```python
from build123d import *

# Parameters (mm, degrees)
F1_DEPTH = 12.7
F4_D     = 13.4874
F5_D     = 25.654


with BuildPart() as f1:
    # F0 (on Front) → F1 (new body)
    with BuildSketch(Plane.XZ):
        with BuildLine():
            Line((-19.05, 50.8), (19.05, 50.8))
            ThreePointArc((19.05, 50.8), (0, 69.85), (-19.05, 50.8))
        make_face()
        with BuildLine():
            ThreePointArc((-19.05, 50.8), (0, 31.75), (19.05, 50.8))
            Line((19.05, 50.8), (-19.05, 50.8))
        make_face()
        with BuildLine():
            ThreePointArc((-19.05, 0), (0, 19.05), (19.05, 0))
            Line((19.05, 0), (19.05, 50.8))
            ThreePointArc((19.05, 50.8), (0, 31.75), (-19.05, 50.8))
            Line((-19.05, 50.8), (-19.05, 0))
        make_face()
        with BuildLine():
            Line((-19.05, 0), (19.05, 0))
            ThreePointArc((19.05, 0), (0, 19.05), (-19.05, 0))
        make_face()
        with BuildLine():
            ThreePointArc((-19.05, 0), (0, -19.05), (19.05, 0))
            Line((19.05, 0), (-19.05, 0))
        make_face()
    extrude(amount=F1_DEPTH)

    # F4 (through all)
    with Locations(Plane.XZ.offset(12.7)):
        with Locations((0, 50.8)):
            Hole(F4_D / 2)

    # F5 (through all)
    with Locations(Plane.XZ.offset(12.7)):
        with Locations((0, 0)):
            Hole(F5_D / 2)


solid = f1.part
```
The listing builds one solid part. Answer for the finished solid, in the listing's coordinates (mm). Give positions to 0.01 mm unless a question says otherwise; leave off trailing zeros. Loops run counter-clockwise (first coordinate to the right, second up) from the corner with the lowest first, then second, coordinate; pieces in that order, holes last. Notation, with made-up numbers: M 80.25,8.25 L 100.25,8.25 A16 ccw 100.25,23.25 Z; hole C -11.75,-27 d11. An arc over 180 degrees is marked long. One line per item, written item: value.
1. Section D-D on x = 9 is taken. Determine the outline of the cut face in (y, z), plus the area to 3 significant figures.
Found:
outline: M -12.7,-16.79 L 0,-16.79 L 0,-9.14 L -12.7,-9.14 Z; M -12.7,9.14 L 0,9.14 L 0,67.59 L -12.7,67.59 Z
area: 839 mm^2
2. Section C-C on z = 3 is taken. Determine the outline of the cut face in (x, y).
Found:
outline: M -19.05,-12.7 L -12.47,-12.7 L -12.47,0 L -19.05,0 Z; M 12.47,-12.7 L 19.05,-12.7 L 19.05,0 L 12.47,0 Z
3. Each of these flat-tipped pins is pushed along its axis until it touches: P1, Ø2, axis at x = -12, y = -10, coming from the +Z side; P2, Ø4, axis at x = 15, y = -5, coming from the +Z side; P3, Ø6, axis at x = -12.5, y = -7, coming from the -Z side. Where does it stop, or does it pass through?
Found:
P1: z = 66.35
P2: z = 64.72
P3: z = -16.51
4. Find the intervals of material crossed by probe 1 along Z at (x, y) = (0.5, -2.5); probe 2 along Z at (x, y) = (3, -10); probe 3 along Z at (x, y) = (-7.5, -8), in increasing order.
Found:
probe 1: -19.04 to -12.82, 12.82 to 44.07, 57.53 to 69.84
probe 2: -18.81 to -12.47, 12.47 to 44.76, 56.84 to 69.61
probe 3: -17.51 to -10.41, 10.41 to 68.31
5. For a pull along Z with two mould halves and no side action, classify faces 1 (the face through (-0.419, -6.261, -19.045)), 2 (the face through (-12.235, -6.261, 3.853)), 3 (the face through (0.878, -6.261, 57.486)), 4 (the face through (0, -12.7, 26)) as pulls with the +Z half, pulls with the -Z half, needs draft (parallel to the pull), parting line crosses it, or undercut.
Found:
face 1: pulls with the -Z half
face 2: undercut
face 3: undercut
face 4: needs draft
6. Section B-B on y = -1.75 is taken. Determine the outline of the cut face in (x, z).
Found:
outline: M -19.05,0 A19.05 ccw 19.05,0 L 19.05,50.8 A19.05 ccw -19.05,50.8 Z; hole C 0,0 d25.65; hole C 0,50.8 d13.49
7. Section A-A on x = 0 is taken. Determine the outline of the cut face in (y, z), plus the area to 3 significant figures.
Found:
outline: M -12.7,-19.05 L 0,-19.05 L 0,-12.83 L -12.7,-12.83 Z; M -12.7,12.83 L 0,12.83 L 0,44.06 L -12.7,44.06 Z; M -12.7,57.54 L 0,57.54 L 0,69.85 L -12.7,69.85 Z
area: 632 mm^2
